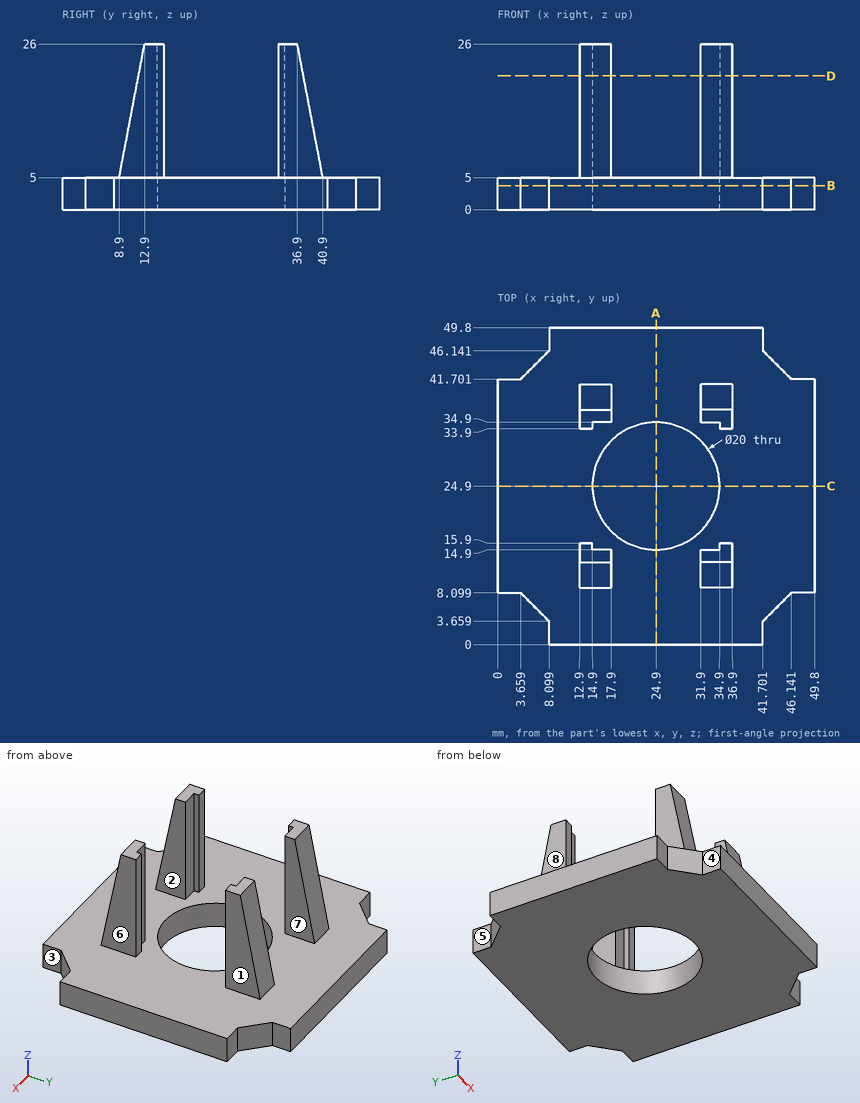
Source: three-view drawing plus pictorial views. Frame: mm from the lowest corner of the part. A direction names the side the tool comes from. Round coordinates to 2 decimals unless told otherwise and drop trailing zeros. Order: outer loops, then holes, each group sorted by start corner. A loop starts at its lowest first (then second) coordinate and runs counter-clockwise, first axis right, second up. Notation, with made-up numbers: M -9.5,67 L 42.5,67 A32 ccw 42.5,100 Z; hole C 9.25,3 d6. An arc over 180 degrees is marked long. One line per item, written item: value.
(1) Cut plane D-D (z = 21). Return the cut outline in (x, y).
Result sheet:
outline: M 12.9,11.95 L 17.9,11.95 L 17.9,14.9 L 14.9,14.9 L 14.9,15.9 L 12.9,15.9 Z; M 12.9,33.9 L 14.9,33.9 L 14.9,34.9 L 17.9,34.9 L 17.9,37.85 L 12.9,37.85 Z; M 31.9,11.95 L 36.9,11.95 L 36.9,15.9 L 34.9,15.9 L 34.9,14.9 L 31.9,14.9 Z; M 31.9,34.9 L 34.9,34.9 L 34.9,33.9 L 36.9,33.9 L 36.9,37.85 L 31.9,37.85 Z
(2) Reachability of the marked faces 1, 2, 3, 4 and 5 from +Z, -Z, +X, -X, +Y, -Y: full face, straight path, thin tool, end or side. Return the list, or none.
Result sheet:
face 1: +Z, +X, +Y, -Y
face 2: +Z, +Y, -Y
face 3: +Z, -Z, +X, -Y
face 4: +Z, -Z, -X, -Y
face 5: +Z, -Z, -X, +Y
(3) Cut plane B-B (z = 3.75). Return the cut outline in (x, y), and give its area (3 significant figures).
Result sheet:
outline: M 0,8.1 L 3.66,8.1 L 8.1,3.66 L 8.1,0 L 41.7,0 L 41.7,3.66 L 46.14,8.1 L 49.8,8.1 L 49.8,41.7 L 46.14,41.7 L 41.7,46.14 L 41.7,49.8 L 8.1,49.8 L 8.1,46.14 L 3.66,41.7 L 0,41.7 Z; hole C 24.9,24.9 d20
area: 1,940 mm2
(4) Pin query (flat end, axial travel): P1, Ø1.5, axis at x = 43.5, y = 13, coming from the +Z side; P2, Ø1, axis at x = 34, z = 16.5, coming from the -Y side (1 decimal); P3, Ø6, axis at y = 15, z = 15, coming from the -X side; P4, Ø6, axis at y = 7.5, z = 17, coming from the +X side. Return the tip coordinate at first contact, or that it passes through.
Result sheet:
P1: z = 5
P2: y = 11
P3: x = 12.9
P4: through
(5) Cut plane A-A (x = 24.9). Return the cut outline in (y, z), and give its area (3 significant figures).
Result sheet:
outline: M 0,0 L 14.9,0 L 14.9,5 L 0,5 Z; M 34.9,0 L 49.8,0 L 49.8,5 L 34.9,5 Z
area: 149 mm2
(6) Pull-direction query (X, two-part tool) for the marked faces 6, 7 and 8; classes: pulls with the +X half, pulls with the -X half, needs draft (parallel to the pull), parting line crosses it, or undercut.
Result sheet:
face 6: pulls with the +X half
face 7: undercut
face 8: pulls with the -X half
(7) Line query: probe 1 along Y at (x, z) = (24.9, 1.4); probe 2 along X at (y, z) = (38, 19.75); probe 3 along Z at (x, y) = (48, 24). Output: solid intervals per line, ascending. Write a range as [from, to].
Result sheet:
probe 1: [0, 14.9], [34.9, 49.8]
probe 2: [12.9, 17.9], [31.9, 36.9]
probe 3: [0, 5]
